from build123d import *

# Parameters (mm, degrees)
SALIENTE_EXTRUIR1_DEPTH = 9
SALIENTE_EXTRUIR2_START = 9
SALIENTE_EXTRUIR2_DEPTH = 30
REDONDEO3_R             = 1
SALIENTE_EXTRUIR3_START = 39
SALIENTE_EXTRUIR3_DEPTH = 8
CORTAR_EXTRUIR1_START   = 47
CROQUIS4_R              = 1.3
CORTAR_EXTRUIR1_DEPTH   = 5
SALIENTE_EXTRUIR4_START = 47
CROQUIS5_R              = 11
CROQUIS5_R_2            = 7.5
SALIENTE_EXTRUIR4_DEPTH = 2
SALIENTE_EXTRUIR5_START = 47
CROQUIS6_R              = 2.5
SALIENTE_EXTRUIR5_DEPTH = 21
CORTAR_EXTRUIR2_START   = 51
CORTAR_EXTRUIR2_DEPTH   = 17
REDONDEO4_R             = 1


with BuildPart() as part:
    # Croquis1 → Saliente-Extruir1 (new body)
    with BuildSketch(Plane(origin=(0, 0, 0), x_dir=(1, 0, 0), z_dir=(0, 1, 0))):
        Polygon((-16.5, 21), (-21, 16.5), (-21, -16.5), (-16.5, -21), (16.5, -21), (21, -16.5), (21, 16.5), (16.5, 21), (8.5, 21), (8.5, 25), (-8.5, 25), (-8.5, 21), align=None)
    extrude(amount=SALIENTE_EXTRUIR1_DEPTH)

    # Croquis2 → Saliente-Extruir2 (add)
    with BuildSketch(Plane(origin=(0, 0, 0), x_dir=(1, 0, 0), z_dir=(0, 1, 0)).offset(SALIENTE_EXTRUIR2_START)):
        Polygon((13, 21), (21, 13), (21, -13), (13, -21), (-13, -21), (-21, -13), (-21, 13), (-13, 21), align=None)
    extrude(amount=SALIENTE_EXTRUIR2_DEPTH)

    # Redondeo3
    redondeo3_edges = [part.edges().sort_by_distance(p)[0] for p in [
        (13, 24, -21),
        (-13, 24, -21),
        (-21, 24, -13),
        (-21, 24, 13),
        (-13, 24, 21),
        (13, 24, 21),
        (21, 24, 13),
        (21, 24, -13),
    ]]
    fillet(redondeo3_edges, radius=REDONDEO3_R)

    # Croquis3 → Saliente-Extruir3 (add)
    with BuildSketch(Plane(origin=(0, 0, 0), x_dir=(1, 0, 0), z_dir=(0, 1, 0)).offset(SALIENTE_EXTRUIR3_START)):
        Polygon((-16.5, 21), (-21, 16.5), (-21, -16.5), (-16.5, -21), (16.5, -21), (21, -16.5), (21, 16.5), (16.5, 21), align=None)
    extrude(amount=SALIENTE_EXTRUIR3_DEPTH)

    # Croquis4 → Cortar-Extruir1 (cut)
    with BuildSketch(Plane(origin=(0, 0, 0), x_dir=(1, 0, 0), z_dir=(0, 1, 0)).offset(CORTAR_EXTRUIR1_START)):
        with Locations(Location((-15.7, 15.7, 0), (0, 0, 270))):
            Circle(CROQUIS4_R)
        with Locations(Location((15.7, 15.7, 0), (0, 0, 270))):
            Circle(CROQUIS4_R)
        with Locations(Location((15.7, -15.7, 0), (0, 0, 270))):
            Circle(CROQUIS4_R)
        with Locations(Location((-15.7, -15.7, 0), (0, 0, 270))):
            Circle(CROQUIS4_R)
    extrude(amount=-CORTAR_EXTRUIR1_DEPTH, mode=Mode.SUBTRACT)

    # Croquis5 → Saliente-Extruir4 (add)
    with BuildSketch(Plane(origin=(0, 0, 0), x_dir=(1, 0, 0), z_dir=(0, 1, 0)).offset(SALIENTE_EXTRUIR4_START)):
        with Locations(Location((0, 0, 0), (0, 0, 90))):
            Circle(CROQUIS5_R)
        with Locations(Location((0, 0, 0), (0, 0, 270))):
            Circle(CROQUIS5_R_2, mode=Mode.SUBTRACT)
    extrude(amount=SALIENTE_EXTRUIR4_DEPTH)

    # Croquis6 → Saliente-Extruir5 (add)
    with BuildSketch(Plane(origin=(0, 0, 0), x_dir=(1, 0, 0), z_dir=(0, 1, 0)).offset(SALIENTE_EXTRUIR5_START)):
        with Locations(Location((0, 0, 0), (0, 0, 90))):
            Circle(CROQUIS6_R)
    extrude(amount=SALIENTE_EXTRUIR5_DEPTH)

    # Croquis7 → Cortar-Extruir2 (cut)
    with BuildSketch(Plane(origin=(0, 0, 0), x_dir=(1, 0, 0), z_dir=(0, 1, 0)).offset(CORTAR_EXTRUIR2_START)):
        with BuildLine():
            Line((2, -1.5), (2, 1.5))
            ThreePointArc((2, 1.5), (2.5, 0), (2, -1.5))
        make_face()
    extrude(amount=CORTAR_EXTRUIR2_DEPTH, mode=Mode.SUBTRACT)

    # Redondeo4
    # the kernel refuses this fillet: 1 mm, written as the material it takes off along each edge
    with BuildSketch(Plane(origin=(0, 68, 0), x_dir=(0, 0, -1), z_dir=(1, 0, 0))) as redondeo4_piece_1:
        with BuildLine():
            CenterArc((2.5 - REDONDEO4_R, -REDONDEO4_R), REDONDEO4_R, 0, 90)
            Line((2.5 - REDONDEO4_R, 0), (2.5, 0))
            Line((2.5, 0), (2.5, -REDONDEO4_R))
        make_face()
    revolve(axis=Axis((0, 68, 0), (0, 1, 0)), revolution_arc=290.580564901, mode=Mode.SUBTRACT)
    with BuildSketch(Plane(origin=(0, 68, 0), x_dir=(0.9370755783657725, 0, 0.34912656792408847), z_dir=(-0.34912656792408847, 0, 0.9370755783657725))) as redondeo4_piece_2:
        with BuildLine():
            CenterArc((2.5 - REDONDEO4_R, -REDONDEO4_R), REDONDEO4_R, 0, 90)
            Line((2.5 - REDONDEO4_R, 0), (2.5, 0))
            Line((2.5, 0), (2.5, -REDONDEO4_R))
        make_face()
    revolve(axis=Axis((0, 68, 0), (0, 1, 0)), revolution_arc=110.433901418, mode=Mode.SUBTRACT)


solid = part.part
The listing builds one solid part. Answer for the finished solid, in the listing's coordinates (mm). A direction names the side the tool comes from. Coordinates: 2 decimals unless noted, no trailing zeros. Write each loop counter-clockwise with the first axis right and the second up, starting at its lowest first coordinate (ties: lowest second). Pieces come first, ordered by that corner, then holes. Notation, with made-up numbers: M -15.75,-32 L -5.75,-32 A24 cw -5.75,-22 Z; hole C -25.75,12.5 d7. An arc over 180 degrees is marked long. Put each result on its own line as item: value. Start each with the question number.
1. A cutting plane is placed at B-B on y = 5.5. Write down the section's boundary in (x, z).
2. Flat-ended cylindrical pins translate along their axes: P1, Ø4, axis at x = 14.5, y = 46.5, coming from the -Z side; P2, Ø10, axis at x = 9.5, y = 54.5, coming from the -Z side; P3, Ø8, axis at x = 16.5, z = -17, coming from the +Y side; P4, Ø1.2, axis at y = 2.5, z = -23, coming from the +X side. Find the tip coordinate at first contact, or state that the pin passes through.
3. A cutting plane is placed at D-D on y = 32. Write down the section's boundary in (x, z), then the cut area to 3 significant figures.
4. For a pull along Y with two mould halves and no side action, classify faces 4 (the flat face through (0, 0, -2)), 5 (the flat face through (-18, 9, 18)), 6 (the flat face through (-18, 9, -18)), 7 (the flat face through (2, 59, 0)) as pulls with the +Y half, pulls with the -Y half, needs draft (parallel to the pull), parting line crosses it, or undercut.
5. Which of the six approach directions +Z, -Z, +X, -X, +Y, -Y give full straight-line access (tool end or side, diameter ignored) to faces 1 (the cylindrical face through (10.74, 47.99, 2.38)), 2 (the flat face through (18, 9, -18)), 3 (the flat face through (18, 9, 18))?
6. Consider line 1 (X direction, y = 45.35, z = 15.7); line 2 (X direction, y = 43, z = -15). Determine where each line is inside the solid, lowest interval first. Write a range as from..to.
7. A cutting plane is placed at C-C on x = -18. Write down the section's boundary in (y, z), then the cut area to 3 significant figures.
8. A cutting plane is placed at A-A on z = -15.7. Write down the section's boundary in (x, y), then the cut area to 3 significant figures.
Resolved:
1. outline: M -21,-16.5 L -16.5,-21 L -8.5,-21 L -8.5,-25 L 8.5,-25 L 8.5,-21 L 16.5,-21 L 21,-16.5 L 21,16.5 L 16.5,21 L -16.5,21 L -21,16.5 Z
2. P1: stops at z = -21
2. P2: passes through
2. P3: stops at y = 47
2. P4: stops at x = 8.5
3. outline: M -21,-12.59 A1 ccw -20.71,-13.29 L -13.29,-20.71 A1 ccw -12.59,-21 L 12.59,-21 A1 ccw 13.29,-20.71 L 20.71,-13.29 A1 ccw 21,-12.59 L 21,12.59 A1 ccw 20.71,13.29 L 13.29,20.71 A1 ccw 12.59,21 L -12.59,21 A1 ccw -13.29,20.71 L -20.71,13.29 A1 ccw -21,12.59 Z
3. area: 1,640 mm2
4. face 4: pulls with the -Y half
4. face 5: undercut
4. face 6: undercut
4. face 7: needs draft
5. face 1: +Y
5. face 2: -Z, +X
5. face 3: +Z, +X
6. line 1: x = -21..-17, -14.4..14.4, 17..21
6. line 2: x = -21..-16.8, -14.6..14.6, 16.8..21
7. outline: M 0,-19.5 L 9,-19.5 L 9,-16 L 39,-16 L 39,-19.5 L 47,-19.5 L 47,19.5 L 39,19.5 L 39,16 L 9,16 L 9,19.5 L 0,19.5 Z
7. area: 1,620 mm2
8. outline: M -21,0 L 21,0 L 21,9 L 18.3,9 L 18.3,39 L 21,39 L 21,47 L 17,47 L 17,42 L 14.4,42 L 14.4,47 L -14.4,47 L -14.4,42 L -17,42 L -17,47 L -21,47 L -21,39 L -18.3,39 L -18.3,9 L -21,9 Z
8. area: 1,790 mm2
